from build123d import *

# Parameters (mm, degrees)
SKETCH1_R           = 108
BOSS_EXTRUDE1_DEPTH = 25
SKETCH2_R           = 108
SKETCH2_R_2         = 100
BOSS_EXTRUDE2_DEPTH = 21
SKETCH3_R           = 50
SKETCH3_R_2         = 27.5
BOSS_EXTRUDE3_DEPTH = 55
SKETCH4_R           = 8
CUT_EXTRUDE1_DEPTH  = 26
SKETCH5_R           = 37.5
CUT_EXTRUDE2_DEPTH  = 6
SKETCH6_R           = 27.5
CUT_EXTRUDE4_DEPTH  = 26
SKETCH7_W           = 16
SKETCH7_H           = 30
CUT_EXTRUDE5_DEPTH  = 81


with BuildPart() as part:
    # Sketch1 → Boss-Extrude1 (new body)
    with BuildSketch(Plane.XY):
        Circle(SKETCH1_R)
    extrude(amount=BOSS_EXTRUDE1_DEPTH)

    # Sketch2 → Boss-Extrude2 (add)
    with BuildSketch(Plane.XY.offset(25)):
        Circle(SKETCH2_R)
        Circle(SKETCH2_R_2, mode=Mode.SUBTRACT)
    extrude(amount=BOSS_EXTRUDE2_DEPTH)

    # Sketch3 → Boss-Extrude3 (add)
    with BuildSketch(Plane.XY.offset(25)):
        Circle(SKETCH3_R)
        Circle(SKETCH3_R_2, mode=Mode.SUBTRACT)
    extrude(amount=BOSS_EXTRUDE3_DEPTH)

    # Sketch4 → Cut-Extrude1 (cut, through all)
    with BuildSketch(Plane.XY.offset(25)):
        with Locations((0, 75)):
            Circle(SKETCH4_R)
        with Locations((75, 0)):
            Circle(SKETCH4_R)
        with Locations((0, -75)):
            Circle(SKETCH4_R)
        with Locations((-75, 0)):
            Circle(SKETCH4_R)
    extrude(amount=-CUT_EXTRUDE1_DEPTH, mode=Mode.SUBTRACT)

    # Sketch5 → Cut-Extrude2 (cut)
    with BuildSketch(Plane(origin=(0, 0, 0), x_dir=(-1, 0, 0), z_dir=(0, 0, -1))):
        Circle(SKETCH5_R)
    extrude(amount=-CUT_EXTRUDE2_DEPTH, mode=Mode.SUBTRACT)

    # Sketch6 → Cut-Extrude4 (cut, through all)
    with BuildSketch(Plane.XY.offset(25)):
        Circle(SKETCH6_R)
    extrude(amount=-CUT_EXTRUDE4_DEPTH, mode=Mode.SUBTRACT)

    # Sketch7 → Cut-Extrude5 (cut, through all)
    with BuildSketch(Plane.XY.offset(80)):
        with Locations((0, 15)):
            Rectangle(SKETCH7_W, SKETCH7_H)
    extrude(amount=-CUT_EXTRUDE5_DEPTH, mode=Mode.SUBTRACT)


solid = part.part
Read the model definition and answer for the solid it produces. Units are mm, in the model's axes. A direction names the side the tool comes from. Round coordinates to 2 decimals unless told otherwise and drop trailing zeros. Write each loop counter-clockwise with the first axis right and the second up, starting at its lowest first coordinate (ties: lowest second). Pieces come first, ordered by that corner, then holes.
Q1. The mould has two halves that part along Y. Classify faces 5 (the face through (46, 2, 0)), 6 (the face through (-23.412, -105.432, 22.678)), 7 (the face through (-46, -21, 25)): released by +Y, released by -Y, zero draft, split by the parting line, or undercut.
Values:
face 5: zero draft
face 6: split by the parting line
face 7: undercut
Q2. Straight lines are drawn through the part: line 1 (Y direction, x = 0, z = 3.8); line 2 (Y direction, x = 0, z = 34.5); line 3 (Z direction, x = -82.5, y = -60). For each, find the intervals that lie inside material, in ascending order.
Values:
line 1: y = -108 to -83, -67 to -37.5, 37.5 to 67, 83 to 108
line 2: y = -108 to -100, -50 to -27.5, 30 to 50, 100 to 108
line 3: z = 0 to 46
Q3. Find section B-B on z = 21.5. Determine the outline of the cut face in (x, y), and give its area (3 significant figures).
Values:
outline: circle Ø216 at (0, 0); hole circle Ø16 at (-75, 0); hole circle Ø16 at (0, -75); hole (-8, 26.31) arc R27.5 ccw (long way) to (8, 26.31) - (8, 30) - (-8, 30) - close; hole circle Ø16 at (0, 75); hole circle Ø16 at (75, 0)
area: 33,400 mm2
Q4. Find section A-A on x = 0. Determine the outline of the cut face in (y, z), and give its area (3 significant figures).
Values:
outline: (-108, 0) - (-83, 0) - (-83, 25) - (-100, 25) - (-100, 46) - (-108, 46) - close; (-67, 0) - (-37.5, 0) - (-37.5, 6) - (-27.5, 6) - (-27.5, 80) - (-50, 80) - (-50, 25) - (-67, 25) - close; (30, 6) - (37.5, 6) - (37.5, 0) - (67, 0) - (67, 25) - (50, 25) - (50, 80) - (30, 80) - close; (83, 0) - (108, 0) - (108, 46) - (100, 46) - (100, 25) - (83, 25) - close
area: 5,730 mm2
Q5. Flat-ended cylindrical pins translate along their axes: P1, Ø5, axis at x = 17.5, z = 9, coming from the +Y side; P2, Ø6, axis at x = -28, z = 18.5, coming from the -Y side; P3, Ø2, axis at x = 11.5, z = 18, coming from the -Y side. Find the tip coordinate at first contact, or state that the pin passes through.
Values:
P1: stops at y = 106.95
P2: stops at y = -105.07
P3: stops at y = -107.49
Q6. A tool of negligible diameter and unlimited length cuts with its end or side. For faces 1 (the face through (-3, -28, 6)), 2 (the face through (22, -22, 80)), 3 (the face through (0, 30, 44)), 4 (the face through (95.38, 30.04, 35.35)), from which of +Z, -Z, +X, -X, +Y, -Y can it reach the whole face along a straight path? Write none if from no direction.
Values:
face 1: -Z
face 2: +Z, +X, -X, +Y, -Y
face 3: +Z, -Z
face 4: +Z
Q7. Find section D-D on z = 73. Determine the outline of the cut face in (x, y).
Values:
outline: circle Ø100 at (0, 0); hole (-8, 26.31) arc R27.5 ccw (long way) to (8, 26.31) - (8, 30) - (-8, 30) - close
Q8. Find section C-C on y = 75. Determine the outline of the cut face in (x, z), and give its area (3 significant figures).
Values:
outline: (-77.71, 0) - (-8, 0) - (-8, 25) - (-66.14, 25) - (-66.14, 46) - (-77.71, 46) - close; (8, 0) - (77.71, 0) - (77.71, 46) - (66.14, 46) - (66.14, 25) - (8, 25) - close
area: 3,970 mm2
